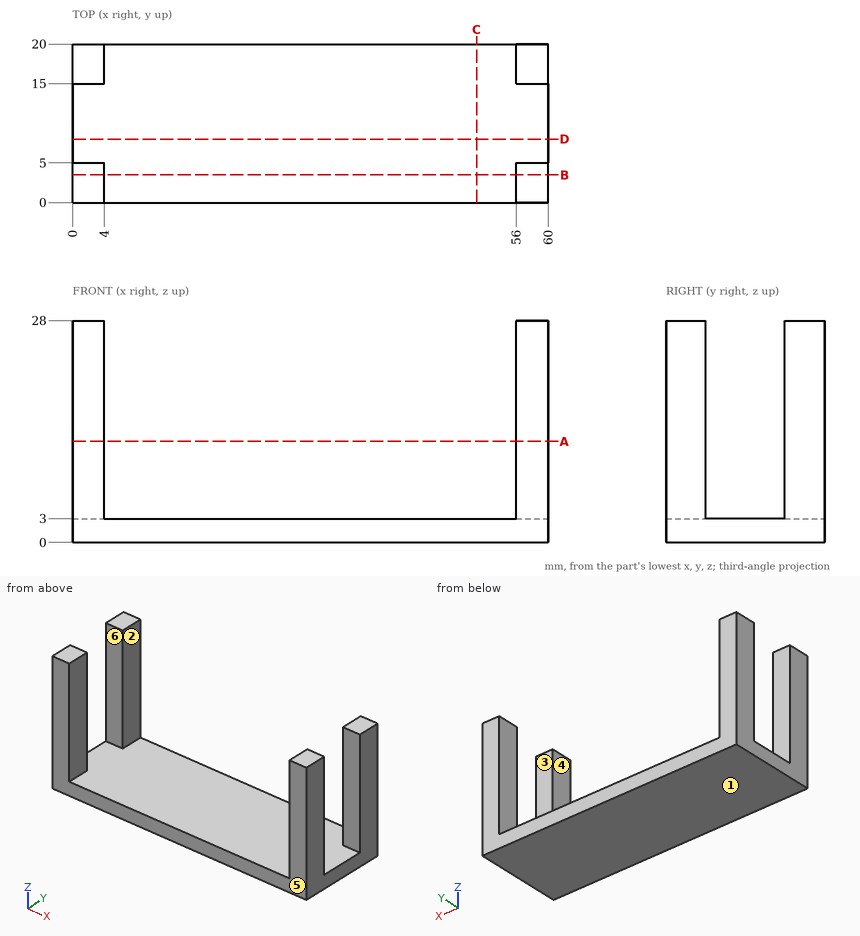
Geometry check sheet. Reference: drawing and pictorial views, mm from the part's lowest x, y, z. A direction names the side the tool comes from. Give positions to 0.01 mm unless a question says otherwise; leave off trailing zeros. Order: outer loops, then holes, each group sorted by start corner. A loop starts at its lowest first (then second) coordinate and runs counter-clockwise, first axis right, second up. Notation, with made-up numbers: M 52.25,35 L 92.25,35 A27 cw 92.25,55 Z; hole C 38.25,3.25 d11. An arc over 180 degrees is marked long. Return JSON: item names as keys, results as strings. Group by question number.
1) Section check B-B on y = 3.5. Record the cut outline in (x, z), and give its area (3 significant figures).
2) Section check A-A on z = 12.75. Record the cut outline in (x, y).
3) Mould release check, pull along Y, two halves, no side actions. Record for the marked faces 4, 5 and 6: pulls with the +Y half, pulls with the -Y half, needs draft (parallel to the pull), parting line crosses it, or undercut.
4) Access from +Z, -Z, +X, -X, +Y, -Y to the whole of each face (thin tool, end or side, straight path). Record for the marked faces 1, 2 and 3.
5) Section check D-D on y = 8. Record the cut outline in (x, z), and give its area (3 significant figures).
6) Section check C-C on x = 51. Record the cut outline in (y, z), and give its area (3 significant figures).
7) Scan lines: line 1 (X direction, y = 4, z = 9); line 2 (Z direction, x = 9, y = 14). Record each from-to range of solid material in increasing order.
8) Go/stop test with flat-tipped pins: pin 1 Ø10 at (x, z) = (8, 10) entering from -Y; pin 2 Ø4 at (x, y) = (21.5, 6) entering from +Z. Record where each tip stops, or that it passes through.
Answer block:
{
 "1": {"outline": "M 0,0 L 60,0 L 60,28 L 56,28 L 56,3 L 4,3 L 4,28 L 0,28 Z", "area": "380 mm^2"},
 "2": {"outline": "M 0,0 L 4,0 L 4,5 L 0,5 Z; M 0,15 L 4,15 L 4,20 L 0,20 Z; M 56,0 L 60,0 L 60,5 L 56,5 Z; M 56,15 L 60,15 L 60,20 L 56,20 Z"},
 "3": {"face 4": "needs draft", "face 5": "pulls with the -Y half", "face 6": "undercut"},
 "4": {"face 1": "-Z, +X, -X, +Y, -Y", "face 2": "+Z, +Y, -Y", "face 3": "+Z, +X, -X"},
 "5": {"outline": "M 0,0 L 60,0 L 60,3 L 0,3 Z", "area": "180 mm^2"},
 "6": {"outline": "M 0,0 L 20,0 L 20,3 L 0,3 Z", "area": "60.0 mm^2"},
 "7": {"line 1": "x = 0 to 4, 56 to 60", "line 2": "z = 0 to 3"},
 "8": {"pin 1": "stops at y = 0", "pin 2": "stops at z = 3"}
}
